Here's how the part is built. I have some questions about the finished solid (model axes, mm). Face numbers are marked on the shaded views. A direction names the side the tool comes from. Round coordinates to 2 decimals unless told otherwise and drop trailing zeros. Order: outer loops, then holes, each group sorted by start corner. A loop starts at its lowest first (then second) coordinate and runs counter-clockwise, first axis right, second up. Notation, with made-up numbers: (83.25, 84.5) -> (110.25, 84.5) arc R9 cw to (110.25, 93.5) -> close; hole circle Ø3 at (10, -5). An arc over 180 degrees is marked (long way). Use a Markdown table: item, result. Add a question column.
(1) I want a section at A-A, the plane z = 6. Please give me the cut outline in (x, y).
(2) On a 3-axis mill with a long thin cutter (end or side, diameter ignored), from which of +Z, -Z, +X, -X, +Y, -Y can I reach the whole of each face in a straight line? I mean the marked faces 4 and 5. Say none if no direction works.
(3) I'm going to push flat-ended pins straight in: P1, Ø12, axis at x = -7, z = 28.5, coming from the -Y side; P2, Ø10, axis at x = -8.5, y = 13, coming from the -Z side; P3, Ø8, axis at y = -16.5, z = 28.5, coming from the -X side. Where does each tip first touch, or does it pass through?
(4) If I drill on probe 1 along X at (y, z) = (0, 8.75); probe 2 along Z at (x, y) = (-13, -28), over which ranges is the centre line in solid material (lowest first)?
(5) Thinking about a two-plate mould opening in X: for the marked faces 1, 2 and 3, which applies, pulls with the +X half, pulls with the -X half, needs draft (parallel to the pull), parting line crosses it, or undercut?
Solid Edge part; units mm, degrees
sketch "Sketch1" plane through (0, 0, 0) normal (0, -1, 0) x (1, 0, 0)
  line L0 (37.5, 0) -> (35.5, 0)
  line L1 (35.5, 0) -> (35.5, 29)
  line L2 (35.5, 29) -> (31.12, 33.38)
  line L3 (31.12, 33.38) -> (0, 33.38)
  line L4 (0, 33.38) -> (0, 35.38)
  line L5 (0, 35.38) -> (32.12, 35.38)
  line L6 (32.12, 35.38) -> (37.5, 30)
  line L7 (37.5, 30) -> (37.5, 0)
  dimension "D1" = 37.5
  dimension "D2" = 37.5
revolve "RevolvedProtrusion1" add sketch "Sketch1" angle 360 about axis through (0, 0, 3.61) along (0, 0, -1)
fillet "Verrundung_1" radius 2 2 edges at (-32.12, 0, 35.38) (-37.5, 0, 30)
properties material "ABS-Plastik, mittlerer Anschlag"
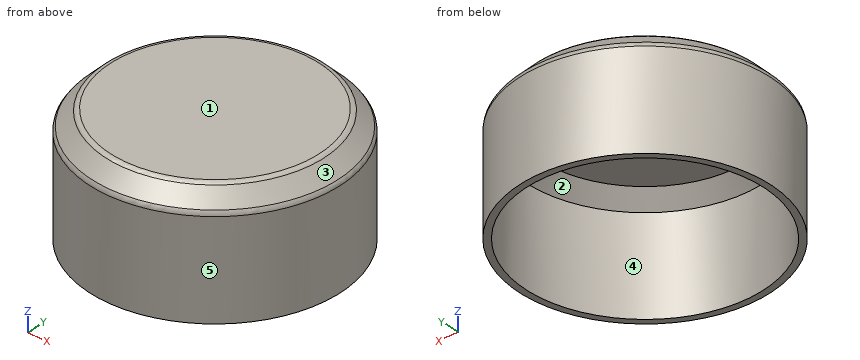
Taken from the geometry:
| question | item | result |
|---|---|---|
| 1 | outline | circle Ø75 at (0, 0); hole circle Ø71 at (0, 0) |
| 2 | face 4 | -Z |
| 2 | face 5 | +Z, -Z |
| 3 | P1 | stops at y = -37.49 |
| 3 | P2 | stops at z = 33.38 |
| 3 | P3 | stops at x = -35.36 |
| 4 | probe 1 | x = -37.5 to -35.5, 35.5 to 37.5 |
| 4 | probe 2 | z = 33.38 to 35.38 |
| 5 | face 1 | needs draft |
| 5 | face 2 | undercut |
| 5 | face 3 | parting line crosses it |
